CAD build for the part. Positions are in the model's coordinates, mm. A direction names the side the tool comes from. Give positions to 0.01 mm unless a question says otherwise; leave off trailing zeros. Loops run counter-clockwise (first coordinate to the right, second up) from the corner with the lowest first, then second, coordinate; pieces in that order, holes last. Notation, with made-up numbers: M 45.25,-9 L 76.25,-9 A30 ccw 76.25,27 Z; hole C -20.75,10.25 d5. An arc over 180 degrees is marked long. Answer as CSV lines item,"result".
```python
from build123d import *

# Parameters (mm, degrees)
BOSS_EXTRUDE1_DEPTH   = 5
BOSS_EXTRUDE1_2_DEPTH = 5
BOSS_EXTRUDE1_3_DEPTH = 5
BOSS_EXTRUDE1_4_DEPTH = 5
SKETCH2_W             = 37.8125
SKETCH2_H             = 39.375
BOSS_EXTRUDE2_DEPTH   = 5
SKETCH3_W             = 55
SKETCH3_H             = 13
SKETCH3_R             = 2.1
BOSS_EXTRUDE3_DEPTH   = 5
SKETCH4_W             = 61
SKETCH4_H             = 30
BOSS_EXTRUDE4_DEPTH   = 5
SKETCH5_R             = 2.5
SKETCH5_W             = 39.983210939
SKETCH5_H             = 20
CUT_EXTRUDE3_DEPTH    = 5
SKETCH7_R             = 2.1
CUT_EXTRUDE4_DEPTH    = 14


with BuildPart() as part:
    # Sketch1 → Boss-Extrude1 (new body)
    with BuildSketch(Plane.XY):
        with BuildLine():
            Line((16.390676557, 6.279692656), (19.828176557, 6.279692656))
            Line((19.828176557, 6.279692656), (19.828176557, 17.279692656))
            Line((19.828176557, 17.279692656), (13.640676557, 17.279692656))
            Line((13.640676557, 17.279692656), (13.640676557, 9.029692656))
            ThreePointArc((13.640676557, 9.029692656), (14.446132909, 7.085149007), (16.390676557, 6.279692656))
        make_face()
    extrude(amount=BOSS_EXTRUDE1_DEPTH)



with BuildPart() as body_2:
    # Sketch1 → Boss-Extrude1 2 (new body)
    with BuildSketch(Plane.XY):
        with BuildLine():
            Line((-17.984323443, 6.279692656), (-14.546823443, 6.279692656))
            ThreePointArc((-14.546823443, 6.279692656), (-12.602279794, 7.085149007), (-11.796823443, 9.029692656))
            Line((-11.796823443, 9.029692656), (-11.796823443, 17.279692656))
            Line((-11.796823443, 17.279692656), (-17.984323443, 17.279692656))
            Line((-17.984323443, 17.279692656), (-17.984323443, 6.279692656))
        make_face()
    extrude(amount=BOSS_EXTRUDE1_2_DEPTH)


with BuildPart() as body_3:
    # Sketch1 → Boss-Extrude1 3 (new body)
    with BuildSketch(Plane.XY):
        with BuildLine():
            Line((19.828176557, -6.095307344), (16.390676557, -6.095307344))
            ThreePointArc((16.390676557, -6.095307344), (14.446132909, -6.900763696), (13.640676557, -8.845307344))
            Line((13.640676557, -8.845307344), (13.640676557, -22.095307344))
            Line((13.640676557, -22.095307344), (19.828176557, -22.095307344))
            Line((19.828176557, -22.095307344), (19.828176557, -6.095307344))
        make_face()
    extrude(amount=BOSS_EXTRUDE1_3_DEPTH)


with BuildPart() as body_4:
    # Sketch1 → Boss-Extrude1 4 (new body)
    with BuildSketch(Plane.XY):
        with BuildLine():
            Line((-11.796823443, -17.095307344), (-11.796823443, -3.845307344))
            ThreePointArc((-11.796823443, -3.845307344), (-12.602279794, -1.900763696), (-14.546823443, -1.095307344))
            Line((-14.546823443, -1.095307344), (-17.984323443, -1.095307344))
            Line((-17.984323443, -1.095307344), (-17.984323443, -17.095307344))
            Line((-17.984323443, -17.095307344), (-11.796823443, -17.095307344))
        make_face()
    extrude(amount=BOSS_EXTRUDE1_4_DEPTH)


with BuildPart() as part_1:
    add(part.part)

    add(body_2.part)  # Boss-Extrude2 merges body 2

    add(body_3.part)  # Boss-Extrude2 merges body 3

    add(body_4.part)  # Boss-Extrude2 merges body 4
    # Sketch2 → Boss-Extrude2 (add)
    with BuildSketch(Plane.XY.offset(5)):
        with Locations((0.921926557, -2.407807344)):
            Rectangle(SKETCH2_W, SKETCH2_H)
    extrude(amount=BOSS_EXTRUDE2_DEPTH)

    # Sketch3 → Boss-Extrude3 (add)
    with BuildSketch(Plane(origin=(0, 17.279692656, 0), x_dir=(1, 0, 0), z_dir=(0, 1, 0))):
        with Locations((9.515676557, -3.5)):
            Rectangle(SKETCH3_W, SKETCH3_H)
        with Locations((-0.484323443, -1)):
            Circle(SKETCH3_R, mode=Mode.SUBTRACT)
        with Locations((19.515676557, -1)):
            Circle(SKETCH3_R, mode=Mode.SUBTRACT)
    boss_extrude3 = extrude(amount=BOSS_EXTRUDE3_DEPTH)

    # Mirror1: Boss-Extrude3 across plane
    add(boss_extrude3.mirror(Plane(origin=(0, -2.407807344, 0), x_dir=(0, 0, 1), z_dir=(0, -1, 0))))

    # Sketch4 → Boss-Extrude4 (add)
    with BuildSketch(Plane(origin=(0, 22.279692656, 0), x_dir=(1, 0, 0), z_dir=(0, 1, 0))):
        with Locations((9.515676557, -25)):
            Rectangle(SKETCH4_W, SKETCH4_H)
    boss_extrude4 = extrude(amount=-BOSS_EXTRUDE4_DEPTH)

    # Mirror2: Boss-Extrude4 across plane
    add(boss_extrude4.mirror(Plane(origin=(0, -2.407807344, 0), x_dir=(0, 0, 1), z_dir=(0, -1, 0))))

    # Sketch5 → Cut-Extrude3 (cut)
    with BuildSketch(Plane.XZ.offset(-17.279692656)):
        with Locations((-23.159015917, 29.025922811)):
            Circle(SKETCH5_R)
        with Locations((-23.159015917, 18.865922811)):
            Circle(SKETCH5_R)
        with Locations((25.840984083, 29.025922811)):
            Circle(SKETCH5_R)
        with Locations((25.840984083, 18.865922811)):
            Circle(SKETCH5_R)
        with Locations((1.332589552, 23.945922811)):
            Rectangle(SKETCH5_W, SKETCH5_H)
    cut_extrude3 = extrude(amount=-CUT_EXTRUDE3_DEPTH, mode=Mode.SUBTRACT)

    # Sketch7 → Cut-Extrude4 (cut, through all)
    with BuildSketch(Plane.XY.offset(10)):
        with Locations((32.015676557, -20.720307344)):
            Circle(SKETCH7_R)
        with Locations((-12.984323443, -20.720307344)):
            Circle(SKETCH7_R)
        with Locations((32.015676557, 5.279692656)):
            Circle(SKETCH7_R)
        with Locations((-12.984323443, 5.279692656)):
            Circle(SKETCH7_R)
    extrude(amount=-CUT_EXTRUDE4_DEPTH, mode=Mode.SUBTRACT)

    # Mirror3: Cut-Extrude3 across plane
    add(cut_extrude3.mirror(Plane(origin=(0, -2.407807344, 0), x_dir=(0, 0, 1), z_dir=(0, -1, 0))), mode=Mode.SUBTRACT)


solid = part_1.part
```
Q1. Wall check: line 1 (X direction, y = -25.6, z = 1); line 2 (Y direction, x = 32, z = 37); line 3 (Z direction, x = -3.5, y = 11.5). Give the ranges that are in metal, low to high. Write a range as [from, to].
Solution:
line 1,"x = [-17.98, -2.58], [1.62, 17.42], [21.62, 37.02]"
line 2,"y = [-27.1, -22.1], [17.28, 22.28]"
line 3,"z = [5, 10]"
Q2. Cut at C-C (x = 14.5). Write the cut outline in (y, z), and give its area (3 significant figures).
Solution:
outline,"M -27.1,-3 L -22.1,-3 L -22.1,0 L -6.85,0 L -6.85,5 L 7.03,5 L 7.03,0 L 17.28,0 L 17.28,-3 L 22.28,-3 L 22.28,13.95 L 17.28,13.95 L 17.28,10 L -22.1,10 L -22.1,13.95 L -27.1,13.95 Z; M -27.1,33.95 L -22.1,33.95 L -22.1,40 L -27.1,40 Z; M 17.28,33.95 L 22.28,33.95 L 22.28,40 L 17.28,40 Z"
area,"554 mm²"
Q3. Mould opens along Y. For faces 1 (the flat face through (19, -22.095, 2)), 2 (the cylindrical face through (-20.66, -24.56, 29.01)), 3 (the flat face through (-15, -17.095, 2)), 4 (the flat face through (-15, -9, 0)) say: released by +Y, released by -Y, zero draft, split by the parting line, or undercut.
Solution:
face 1,"released by -Y"
face 2,"zero draft"
face 3,"undercut"
face 4,"undercut"
Q4. Which spindle directions (+Z, -Z, +X, -X, +Y, -Y) get a long thin tool onto all of the face, cutting with end or side? Do faces 5 (the cylindrical face through (21.52, 19.74, 0.37)), 6 (the cylindrical face through (-20.66, 19.74, 29.01)), 7 (the flat face through (18, 6.28, 2)), 8 (the flat face through (38, 20, 10)), 9 (the flat face through (1, -25, 33.946)). Say none if no direction does.
Solution:
face 5,"+Y"
face 6,"-X, +Y, -Y"
face 7,"-Z, +X, -X"
face 8,"-Z, +X, +Y, -Y"
face 9,"+Y, -Y"
Q5. Cut at D-D (z = 1). Give the number of separate pieces and of enclosed holes in the cut face, and give its area (3 significant figures).
Solution:
separate pieces,"7"
enclosed holes,"0"
area,"789 mm²"
Q6. Cut at B-B (y = -10). Write the cut outline in (x, z), and give its area (3 significant figures).
Solution:
outline,"M -17.98,0 L -11.8,0 L -11.8,5 L 13.64,5 L 13.64,0 L 19.83,0 L 19.83,10 L -17.98,10 Z"
area,"251 mm²"
Q7. Pin check, flat tips, straight feed: P1, Ø12, axis at x = 1.5, y = -7.5, coming from the +Z side; P2, Ø3, axis at y = 16, z = 15, coming from the -X side; P3, Ø2.5, axis at y = -9.5, z = 3.5, coming from the +X side; P4, Ø1.5, axis at x = 38.5, y = -24.5, coming from the -Z side. Stop position of each tip, or through.
Solution:
P1,"stops at z = 10"
P2,"stops at x = -20.98"
P3,"stops at x = 19.83"
P4,"stops at z = 10"
Q8. Cut at A-A (z = 15.5). Write the cut outline in (x, y).
Solution:
outline,"M -20.98,-27.1 L -18.66,-27.1 L -18.66,-22.1 L -20.98,-22.1 Z; M -20.98,17.28 L -18.66,17.28 L -18.66,22.28 L -20.98,22.28 Z; M 21.32,-27.1 L 40.02,-27.1 L 40.02,-22.1 L 21.32,-22.1 Z; M 21.32,17.28 L 40.02,17.28 L 40.02,22.28 L 21.32,22.28 Z"
